Source: CAD feature listing. Evaluate the final solid. Frame: model axes, mm. Give positions to 0.01 mm unless a question says otherwise; leave off trailing zeros. Write each loop counter-clockwise with the first axis right and the second up, starting at its lowest first coordinate (ties: lowest second). Pieces come first, ordered by that corner, then holes. Notation, with made-up numbers: (38.25, 61) -> (61.25, 61) arc R16 cw to (61.25, 91) -> close; hole circle Ø6 at (72, 58). An arc over 180 degrees is marked (long way). Answer as a JSON object with one key per item and string values. Group by question number.
Item 1: Section query C-C on z = 3.5. Give the number of separate pieces and of enclosed holes in the cut face, plus the area to 3 significant figures.
Item 2: First-contact query: pin 1 Ø3 at (x, y) = (53, 9.5) entering from -Z. Flat tip, straight axial feed; report the tip coordinate or a pass-through.
Item 3: Section query B-B on y = 15. Return the cut outline in (x, z), plus the area to 3 significant figures.
Item 4: Section query A-A on x = 30.5. Return the cut outline in (y, z) (3 decimals), plus the area to 3 significant figures.
Item 5: Ray query, probe 1 along X at (y, z) = (31.5, 2.5); probe 2 along X at (y, z) = (35.5, 3.75); probe 3 along Y at (x, z) = (28, 6) (3 decimals). Return the intervals inside material, ascending. Write a range as from..to.
Item 6: Pull-direction query (X, two-part tool) for faces 1 (the face through (12.7, 24, 3)), 2 (the face through (44, 3.175, 3)), 3 (the face through (67.844, 32.413, 3.131)); classes: pulls with the +X half, pulls with the -X half, needs draft (parallel to the pull), parting line crosses it, or undercut.
from build123d import *

# Parameters (mm, degrees)
SKETCH1_W               = 63.5
SKETCH1_H               = 41.275
BOSS_EXTRUDE1_DEPTH     = 6.35
CUT_EXTRUDE1_DEPTH      = 89.44526556
CUT_EXTRUDE1_DEPTH_BACK = 89.44526556
SKETCH3_R               = 2.413
FILLET1_SIZE            = 3.175


with BuildPart() as part:
    # Sketch1 → Boss-Extrude1 (new body)
    with BuildSketch(Plane.XY):
        with Locations((44.45, 23.8125)):
            Rectangle(SKETCH1_W, SKETCH1_H)
    extrude(amount=BOSS_EXTRUDE1_DEPTH)

    # Sketch3 → Cut-Extrude1 (cut, two sides: drawn at the far end of the back side and taken through both)
    with BuildSketch(Plane.XY.offset(6.35).offset(-CUT_EXTRUDE1_DEPTH_BACK)):
        with Locations((65.615475516, 33.3375)):
            Circle(SKETCH3_R)
        with Locations((28.785475516, 33.3375)):
            Circle(SKETCH3_R)
        with Locations((28.785475516, 14.2875)):
            Circle(SKETCH3_R)
        with Locations((65.615475516, 14.2875)):
            Circle(SKETCH3_R)
    extrude(amount=CUT_EXTRUDE1_DEPTH + CUT_EXTRUDE1_DEPTH_BACK, mode=Mode.SUBTRACT)

    # Fillet1
    # a fillet whose section is not a circle: 3.175 mm, written as the material it takes off along each edge
    with BuildSketch(Plane(origin=(12.7, 3.175, -7.9375), x_dir=(1, 0, 0), z_dir=(0, 0, 1)), Plane(origin=(12.7, 44.45, -7.9375), x_dir=(0, -1, 0), z_dir=(0, 0, 1))) as fillet1_piece_1:
        with BuildLine():
            add(Edge.make_bspline([(FILLET1_SIZE, 0), (FILLET1_SIZE * 0.831801948466, 0), (FILLET1_SIZE * 0.663603896932, 0), (FILLET1_SIZE * 0.292893218813, FILLET1_SIZE * 0.0716919198361), (FILLET1_SIZE * 0.0716919198361, FILLET1_SIZE * 0.292893218813), (0, FILLET1_SIZE * 0.663603896932), (0, FILLET1_SIZE * 0.831801948466), (0, FILLET1_SIZE)], knots=[0, 0, 0, 0, 0, 0, 0.5, 0.5, 1, 1, 1, 1, 1, 1], degree=5))
            Line((0, FILLET1_SIZE), (0, 0))
            Line((0, 0), (FILLET1_SIZE, 0))
        make_face()
    extrude(amount=22.225, mode=Mode.SUBTRACT)
    with BuildSketch(Plane(origin=(76.2, 3.175, -7.9375), x_dir=(-1, 0, 0), z_dir=(0, 0, 1)), Plane(origin=(76.2, 44.45, -7.9375), x_dir=(0, -1, 0), z_dir=(0, 0, 1))) as fillet1_piece_2:
        with BuildLine():
            add(Edge.make_bspline([(FILLET1_SIZE, 0), (FILLET1_SIZE * 0.831801948466, 0), (FILLET1_SIZE * 0.663603896932, 0), (FILLET1_SIZE * 0.292893218813, -FILLET1_SIZE * 0.0716919198361), (FILLET1_SIZE * 0.0716919198361, -FILLET1_SIZE * 0.292893218813), (0, -FILLET1_SIZE * 0.663603896932), (0, -FILLET1_SIZE * 0.831801948466), (0, -FILLET1_SIZE)], knots=[0, 0, 0, 0, 0, 0, 0.5, 0.5, 1, 1, 1, 1, 1, 1], degree=5))
            Line((0, -FILLET1_SIZE), (0, 0))
            Line((0, 0), (FILLET1_SIZE, 0))
        make_face()
    extrude(amount=22.225, mode=Mode.SUBTRACT)


solid = part.part
Worked answers:
{
 "1": {"separate pieces": "1", "enclosed holes": "4", "area": "2,540 mm^2"},
 "2": {"pin 1": "z = 0"},
 "3": {"outline": "(12.7, 0) -> (26.48, 0) -> (26.48, 6.35) -> (12.7, 6.35) -> close; (31.09, 0) -> (63.31, 0) -> (63.31, 6.35) -> (31.09, 6.35) -> close; (67.92, 0) -> (76.2, 0) -> (76.2, 6.35) -> (67.92, 6.35) -> close", "area": "345 mm^2"},
 "4": {"outline": "(3.175, 0) -> (12.59, 0) -> (12.59, 6.35) -> (3.175, 6.35) -> close; (15.985, 0) -> (31.64, 0) -> (31.64, 6.35) -> (15.985, 6.35) -> close; (35.035, 0) -> (44.45, 0) -> (44.45, 6.35) -> (35.035, 6.35) -> close", "area": "219 mm^2"},
 "5": {"probe 1": "12.7..27.22, 30.35..64.05, 67.18..76.2", "probe 2": "12.7..27.71, 29.86..64.54, 66.69..76.2", "probe 3": "3.175..12.006, 16.569..31.056, 35.619..44.45"},
 "6": {"face 1": "pulls with the -X half", "face 2": "needs draft", "face 3": "undercut"}
}
